Design review of the part built by this model. Coordinates are the model's own, in mm. Give positions to 0.01 mm unless a question says otherwise; leave off trailing zeros. Write each loop counter-clockwise with the first axis right and the second up, starting at its lowest first coordinate (ties: lowest second). Pieces come first, ordered by that corner, then holes. Notation, with made-up numbers: (-32, -5) -> (-25, -5) arc R20 ccw to (-25, 29) -> close; hole circle Ø3 at (-28.5, 42). An arc over 180 degrees is marked (long way). Put each result on its own line as item: value. Start each with the question number.
Autodesk Inventor part; units mm, degrees
ref_plane "YZ Plane" through (0, 0, 0) normal (1, 0, 0) x (0, 1, 0)
ref_plane "XZ Plane" through (0, 0, 0) normal (0, 1, 0) x (-1, 0, 0)
ref_plane "XY Plane" through (0, 0, 0) normal (0, 0, 1) x (1, 0, 0)
sketch "Sketch1" plane through (0, 0, 0) normal (0, 0, 1) x (1, 0, 0)
  circle A0 centre (13, 0) radius 1.5
  circle A1 centre (6.5, 11.2583) radius 1.5
  arc A2 (9.9641, 13.2583) -> (3.0359, 13.2583) centre (6.5, 11.2583) ccw
  arc A3 (13, -4) -> (16.4641, 2) centre (13, 0) ccw
  line L0 (9.9641, 13.2583) -> (16.4641, 2)
  arc A4 (3.2, -2.4) -> (-0.4785, 3.9713) centre (0, 0) ccw
  line L1 (4, -4) -> (13, -4)
  line L2 (-1.4641, 5.4641) -> (3.0359, 13.2583)
  arc A5 (-1.4641, 5.4641) -> (-0.4785, 3.9713) centre (-0.5981, 4.9641) ccw
  arc A6 (3.2, -2.4) -> (4, -4) centre (4, -3) ccw
  point P0 (0, -4)
  point P1 (-3.4641, 2)
  dimension "d0" = 3
  dimension "d1" = 3
  dimension "d3" = 13
  dimension "d4" = 13
  dimension "d24" = 60
  dimension "d25" = 8
  dimension "d26" = 8
  dimension "d27" = 8
  dimension "d30" = 1
extrude "Extrusion1" add sketch "Sketch1" along normal blind 6
properties part number "X_zaslepka"
Q1. Take a section at D-D on x = 10.5. Give the boundary of the cut face in (y, z), then the cut area to 3 significant figures.
Q2. Take a section at B-B on y = 0. Give the boundary of the cut face in (x, z).
Q3. Mouldability with a two-part tool opening along Y and no side actions: class faces 1 (the face through (5.394, 10.245, 2.958)), 2 (the face through (8, 4, 6)), 3 (the face through (6.441, 15.258, 2.958)), 4 (the face through (-1.424, 4.4, 2.958)) as +Y half, -Y half, draft (parallel to the pull), parting line (faces both ways), or undercut.
Q4. Take a section at C-C on z = 5.4. Give the boundary of the cut face in (x, y), then the cut area to 3 significant figures.
Q5. For pin 1 (3 mm diameter, centred on x = 15, z = 2.5, fed in from -Y); pin 2 (1 mm diameter, centred on y = 11.5, z = 2, fed in from -X); pin 3 (1.5 mm diameter, centred on y = 11.5, z = 1, fed in from +X), all flat-tipped, find the tip position at first contact; note any pin that passes through.
Q6. Take a section at A-A on x = 6.5. Give the boundary of the cut face in (y, z).
Q7. To check wall thickness, follow probe 1 along Y at (x, z) = (6.5, 1.9); probe 2 along Y at (x, z) = (13, 1.7); probe 3 along X at (y, z) = (0.75, 2.6). State the ranges of each line that lie inside material, in increasing order. Write a range as from..to.
Result:
1. outline: (-4, 0) -> (12.33, 0) -> (12.33, 6) -> (-4, 6) -> close
1. area: 98.0 mm^2
2. outline: (4, 0) -> (11.5, 0) -> (11.5, 6) -> (4, 6) -> close; (14.5, 0) -> (17, 0) -> (17, 6) -> (14.5, 6) -> close
3. face 1: undercut
3. face 2: draft
3. face 3: +Y half
3. face 4: parting line
4. outline: (-1.46, 5.46) arc R1 ccw to (-0.48, 3.97) arc R4 cw to (3.2, -2.4) arc R1 ccw to (4, -4) -> (13, -4) arc R4 ccw to (16.46, 2) -> (9.96, 13.26) arc R4 ccw to (3.04, 13.26) -> close; hole circle Ø3 at (6.5, 11.26); hole circle Ø3 at (13, 0)
4. area: 212 mm^2
5. pin 1: stops at y = -3.97
5. pin 2: stops at x = 1.73
5. pin 3: stops at x = 11.41
6. outline: (-4, 0) -> (9.76, 0) -> (9.76, 6) -> (-4, 6) -> close; (12.76, 0) -> (15.26, 0) -> (15.26, 6) -> (12.76, 6) -> close
7. probe 1: y = -4..9.76, 12.76..15.26
7. probe 2: y = -4..-1.5, 1.5..8
7. probe 3: x = 3.93..11.7, 14.3..16.93
